from build123d import *

# Parameters (mm, degrees)
SKETCH1_W           = 60
SKETCH1_H           = 10
BOSS_EXTRUDE1_DEPTH = 3
SKETCH2_R           = 2
CUT_EXTRUDE1_DEPTH  = 3
SKETCH3_W           = 3
SKETCH3_H           = 6
CUT_EXTRUDE2_DEPTH  = 3
FILLET1_R           = 3


with BuildPart() as part:
    # Sketch1 → Boss-Extrude1 (new body)
    with BuildSketch(Plane.XY):
        Rectangle(SKETCH1_W, SKETCH1_H)
    extrude(amount=BOSS_EXTRUDE1_DEPTH)

    # Sketch2 → Cut-Extrude1 (cut)
    with BuildSketch(Plane.XY.offset(3)):
        Circle(SKETCH2_R)
    extrude(amount=-CUT_EXTRUDE1_DEPTH, mode=Mode.SUBTRACT)

    # Sketch3 → Cut-Extrude2 (cut)
    with BuildSketch(Plane.XY.offset(3)):
        with Locations((-25.5, 0)):
            Rectangle(SKETCH3_W, SKETCH3_H)
    cut_extrude2 = extrude(amount=-CUT_EXTRUDE2_DEPTH, mode=Mode.SUBTRACT)

    # Mirror1: Cut-Extrude2 across plane
    add(cut_extrude2.mirror(Plane(origin=(0, 0, 0), x_dir=(0, 0, 1), z_dir=(1, 0, 0))), mode=Mode.SUBTRACT)

    # Fillet1
    fillet1_edges = [part.edges().sort_by_distance(p)[0] for p in [
        (30, -5, 1.5),
        (-30, -5, 1.5),
        (-30, 5, 1.5),
        (30, 5, 1.5),
    ]]
    fillet(fillet1_edges, radius=FILLET1_R)


solid = part.part
Here's how the part is built. I have some questions about the finished solid (model axes, mm). A direction names the side the tool comes from. Coordinates: 2 decimals unless noted, no trailing zeros. Loops run counter-clockwise (first coordinate to the right, second up) from the corner with the lowest first, then second, coordinate; pieces in that order, holes last. Notation, with made-up numbers: (81, -19.5) -> (137, -19.5) arc R16 ccw to (137, 4.5) -> close; hole circle Ø5 at (29.5, 80.25). An arc over 180 degrees is marked (long way). Use one line per item in the form item = value. Start each with the question number.
(1) If we section it at D-D (x = 0): Please give me the cut outline in (y, z).
(2) If we section it at A-A (x = -25): Please give me the cut outline in (y, z).
(3) On a 3-axis mill with a long thin cutter (end or side, diameter ignored), from which of +Z, -Z, +X, -X, +Y, -Y can I reach the whole of each face in a straight line? I mean faces 5 (the face through (-30, 0, 1)), 6 (the face through (-26, 3, 2)). Say none if no direction works.
(4) If we section it at C-C (z = 1.1): Please give me the cut outline in (x, y).
(5) If we section it at B-B (y = 0): Please give me the cut outline in (x, z), then the cut area to 3 significant figures.
(6) Please list where these lines run through material, in increasing order: line 1 along X through (y, z) = (-0.5, 2.8); line 2 along Y through (x, z) = (0, 0.9); line 3 along Y through (x, z) = (-24.5, 1.55).
(7) We'd pull the mould along Y, two halves only. Please class faces 1 (the face through (-0.4, 2.3, 3)), 2 (the face through (-27, 0, 2)), 3 (the face through (0, 5, 1)), 4 (the face through (0, -2, 2)): pulls with the +Y half, pulls with the -Y half, needs draft (parallel to the pull), parting line crosses it, or undercut.
(8) Will this pin go through, and if not, where does the flat tip stop? pin 1 (5 mm diameter, centred on x = -19.5, y = -0.5, fed in from -Z).
Verdict:
q1.outline = (-5, 0) -> (-2, 0) -> (-2, 3) -> (-5, 3) -> close; (2, 0) -> (5, 0) -> (5, 3) -> (2, 3) -> close
q2.outline = (-5, 0) -> (-3, 0) -> (-3, 3) -> (-5, 3) -> close; (3, 0) -> (5, 0) -> (5, 3) -> (3, 3) -> close
q3.face_5 = +Z, -Z, -X, +Y, -Y
q3.face_6 = +Z, -Z
q4.outline = (-30, -2) arc R3 ccw to (-27, -5) -> (27, -5) arc R3 ccw to (30, -2) -> (30, 2) arc R3 ccw to (27, 5) -> (-27, 5) arc R3 ccw to (-30, 2) -> close; hole (-27, -3) -> (-24, -3) -> (-24, 3) -> (-27, 3) -> close; hole circle Ø4 at (0, 0); hole (24, -3) -> (27, -3) -> (27, 3) -> (24, 3) -> close
q5.outline = (-30, 0) -> (-27, 0) -> (-27, 3) -> (-30, 3) -> close; (-24, 0) -> (-2, 0) -> (-2, 3) -> (-24, 3) -> close; (2, 0) -> (24, 0) -> (24, 3) -> (2, 3) -> close; (27, 0) -> (30, 0) -> (30, 3) -> (27, 3) -> close
q5.area = 150 mm²
q6.line_1 = -30 to -27, -24 to -1.94, 1.94 to 24, 27 to 30
q6.line_2 = -5 to -2, 2 to 5
q6.line_3 = -5 to -3, 3 to 5
q7.face_1 = needs draft
q7.face_2 = undercut
q7.face_3 = pulls with the +Y half
q7.face_4 = undercut
q8.pin_1 = 0
